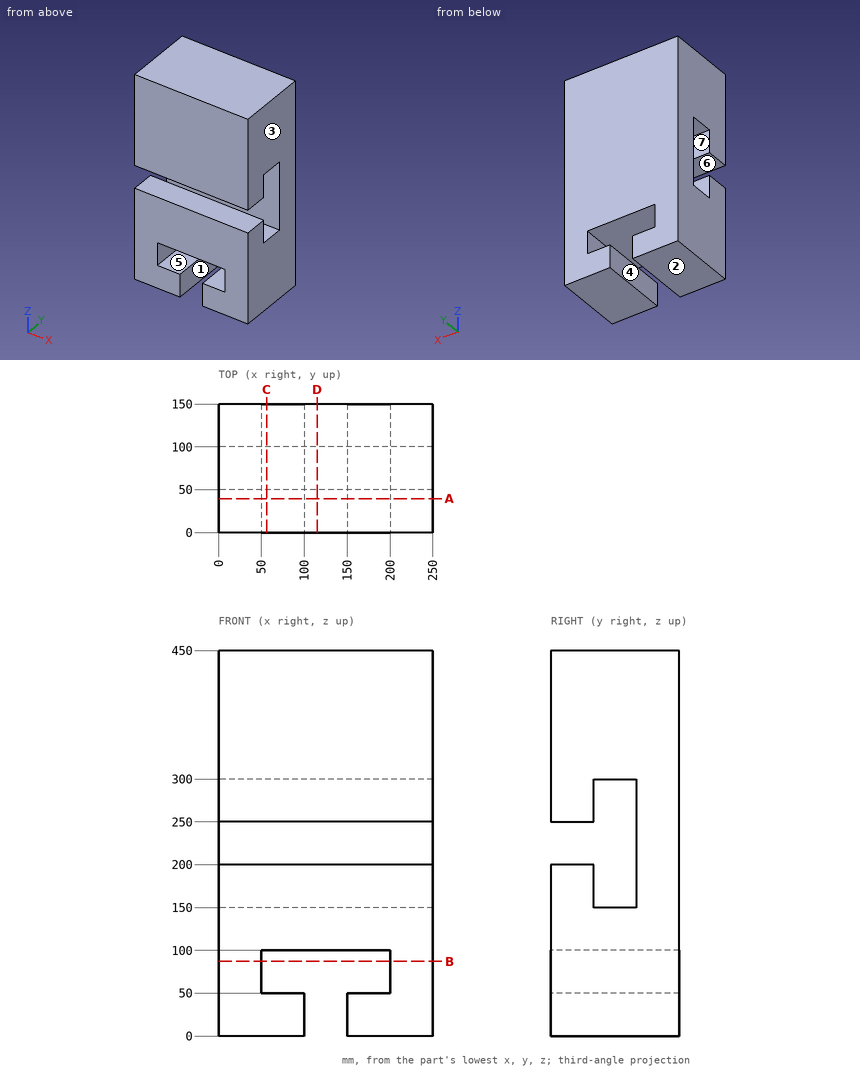
Geometry check sheet. Reference: drawing and pictorial views, mm from the part's lowest x, y, z. A direction names the side the tool comes from. Round coordinates to 2 decimals unless told otherwise and drop trailing zeros. Loops run counter-clockwise (first coordinate to the right, second up) from the corner with the lowest first, then second, coordinate; pieces in that order, holes last. Notation, with made-up numbers: M 12,-18 L 64,-18 A25 cw 64,7 Z; hole C 84.25,-35.75 d2. An arc over 180 degrees is marked long. Return JSON: item names as keys, results as strings. Group by question number.
(1) Set-up check for the marked faces 4, 5, 6 and 7: record each of +Z, -Z, +X, -X, +Y, -Y from which the full face is reachable in a straight line by a thin tool's end or side.
(2) Section check D-D, the plane x = 115. Enter the section's corners in (y, z).
(3) Section check A-A, the plane y = 39.5. Enter the section's corners in (x, z), and give its area (3 significant figures).
(4) Section check B-B, the plane z = 87. Enter the section's corners in (x, y), and give its area (3 significant figures).
(5) Scan lines: line 1 along Z through (x, y) = (183, 87); line 2 along Y through (x, z) = (47.5, 263); line 3 along Z through (x, y) = (231.5, 49.5). Record each from-to range of solid material in increasing order. Write a range as [from, to].
(6) Mould release check, pull along X, two halves, no side actions. Record for the marked faces 1, 2 and 3: pulls with the +X half, pulls with the -X half, needs draft (parallel to the pull), parting line crosses it, or undercut.
(7) Section check C-C, the plane x = 56. Enter the section's corners in (y, z), and give its area (3 significant figures).
Data:
{
 "1": {"face 4": "-Z, +Y, -Y", "face 5": "+Y, -Y", "face 6": "+X, -X, -Y", "face 7": "+X, -X"},
 "2": {"outline": "M 0,100 L 150,100 L 150,450 L 0,450 L 0,250 L 50,250 L 50,300 L 100,300 L 100,150 L 50,150 L 50,200 L 0,200 Z"},
 "3": {"outline": "M 0,0 L 100,0 L 100,50 L 50,50 L 50,100 L 200,100 L 200,50 L 150,50 L 150,0 L 250,0 L 250,200 L 0,200 Z; M 0,250 L 250,250 L 250,450 L 0,450 Z", "area": "90,000 mm²"},
 "4": {"outline": "M 0,0 L 50,0 L 50,150 L 0,150 Z; M 200,0 L 250,0 L 250,150 L 200,150 Z", "area": "15,000 mm²"},
 "5": {"line 1": "[0, 50], [100, 150], [300, 450]", "line 2": "[0, 50], [100, 150]", "line 3": "[0, 200], [250, 450]"},
 "6": {"face 1": "undercut", "face 2": "needs draft", "face 3": "pulls with the +X half"},
 "7": {"outline": "M 0,0 L 150,0 L 150,50 L 0,50 Z; M 0,100 L 150,100 L 150,450 L 0,450 L 0,250 L 50,250 L 50,300 L 100,300 L 100,150 L 50,150 L 50,200 L 0,200 Z", "area": "50,000 mm²"}
}
